Part print with two shaded views. Sizes in mm from the minimum x, y, z corner. A direction names the side the tool comes from. Give positions to 0.01 mm unless a question says otherwise; leave off trailing zeros. Order: outer loops, then holes, each group sorted by start corner. A loop starts at its lowest first (then second) coordinate and runs counter-clockwise, first axis right, second up. Notation, with made-up numbers: (40.25, -37.5) -> (66.25, -37.5) arc R11 ccw to (66.25, -31.5) -> close; hole circle Ø7 at (50, 28.5). An arc over 180 degrees is marked (long way). Answer in a Markdown table with one row per item. Add a question column.
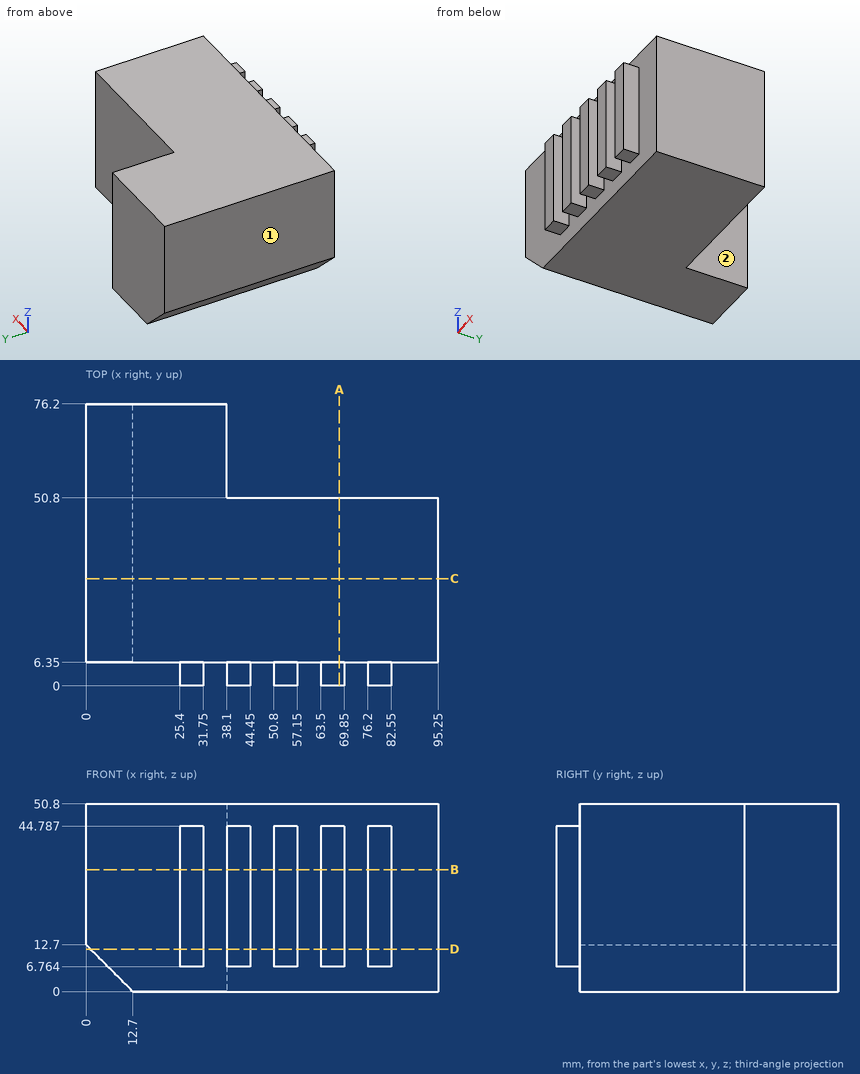
Item 1: Wall check: line 1 (Y direction, x = 12.5, z = 27); line 2 (Y direction, x = 75.5, z = 30.5); line 3 (Z direction, x = 78.5, y = 5.5). Give the ranges that are in metal, low to high.
Item 2: Saw through at C-C on y = 29. List the corners of the cut face in (x, z).
Item 3: Pin check, flat tips, straight feed: pin 1 Ø5 at (y, z) = (3, 34) entering from +X; pin 2 Ø1.5 at (x, z) = (63.5, 31) entering from +Y; pin 3 Ø5 at (x, y) = (27.5, 3) entering from +Z. Stop position of each tip, or through.
Item 4: Saw through at B-B on z = 33. List the corners of the cut face in (x, y), plus the area to 3 significant figures.
Item 5: Which spindle directions (+Z, -Z, +X, -X, +Y, -Y) get a long thin tool onto all of the face, cutting with end or side? Do the marked faces 1 and 2. Say none if no direction does.
Item 6: Saw through at D-D on z = 11.5. List the corners of the cut face in (x, y), plus the area to 3 significant figures.
Item 7: Saw through at A-A on x = 68.5. List the corners of the cut face in (y, z).
Evaluation:
| question | item | result |
|---|---|---|
| 1 | line 1 | y = 6.35 to 76.2 |
| 1 | line 2 | y = 6.35 to 50.8 |
| 1 | line 3 | z = 6.76 to 44.79 |
| 2 | outline | (0, 12.7) -> (12.7, 0) -> (95.25, 0) -> (95.25, 50.8) -> (0, 50.8) -> close |
| 3 | pin 1 | stops at x = 82.55 |
| 3 | pin 2 | stops at y = 50.8 |
| 3 | pin 3 | stops at z = 44.79 |
| 4 | outline | (0, 6.35) -> (25.4, 6.35) -> (25.4, 0) -> (31.75, 0) -> (31.75, 6.35) -> (38.1, 6.35) -> (38.1, 0) -> (44.45, 0) -> (44.45, 6.35) -> (50.8, 6.35) -> (50.8, 0) -> (57.15, 0) -> (57.15, 6.35) -> (63.5, 6.35) -> (63.5, 0) -> (69.85, 0) -> (69.85, 6.35) -> (76.2, 6.35) -> (76.2, 0) -> (82.55, 0) -> (82.55, 6.35) -> (95.25, 6.35) -> (95.25, 50.8) -> (38.1, 50.8) -> (38.1, 76.2) -> (0, 76.2) -> close |
| 4 | area | 5,400 mm2 |
| 5 | face 1 | +Z, -Z, -X, +Y, -Y |
| 5 | face 2 | +Z, -Z, +X, +Y |
| 6 | outline | (1.2, 6.35) -> (25.4, 6.35) -> (25.4, 0) -> (31.75, 0) -> (31.75, 6.35) -> (38.1, 6.35) -> (38.1, 0) -> (44.45, 0) -> (44.45, 6.35) -> (50.8, 6.35) -> (50.8, 0) -> (57.15, 0) -> (57.15, 6.35) -> (63.5, 6.35) -> (63.5, 0) -> (69.85, 0) -> (69.85, 6.35) -> (76.2, 6.35) -> (76.2, 0) -> (82.55, 0) -> (82.55, 6.35) -> (95.25, 6.35) -> (95.25, 50.8) -> (38.1, 50.8) -> (38.1, 76.2) -> (1.2, 76.2) -> close |
| 6 | area | 5,320 mm2 |
| 7 | outline | (0, 6.76) -> (6.35, 6.76) -> (6.35, 0) -> (50.8, 0) -> (50.8, 50.8) -> (6.35, 50.8) -> (6.35, 44.79) -> (0, 44.79) -> close |
